The listing builds one solid part. Answer for the finished solid, in the listing's coordinates (mm). Face numbers are marked on the shaded views. A direction names the side the tool comes from. Give positions to 0.01 mm unless a question says otherwise; leave off trailing zeros. Write each loop counter-clockwise with the first axis right and the second up, starting at its lowest first coordinate (ties: lowest second). Pieces come first, ordered by that corner, then holes. Notation, with made-up numbers: M 85,27 L 116,27 A18 cw 116,45 Z; hole C -39.5,-23.75 d11. An arc over 180 degrees is marked long. Return JSON: item names as keys, results as strings.
from build123d import *

# Parameters (mm, degrees)
LINEAR_AUSTRAGEN_D_NN1_DEPTH    = 20
FASE1_SIZE                      = 1
SKIZZE2_R                       = 1.5
SCHNITT_LINEAR_AUSTRAGEN1_DEPTH = 10
SKIZZE3_R                       = 1.5
SCHNITT_LINEAR_AUSTRAGEN2_DEPTH = 10
SKIZZE4_R                       = 2.25
SCHNITT_LINEAR_AUSTRAGEN3_DEPTH = 10


with BuildPart() as part:
    # Skizze1 → Linear-Austragen-Dünn1 (new, symmetric)
    with BuildSketch(Plane.XY):
        Polygon((0, 10), (0, 0), (10, 0), (10, 1), (1, 1), (1, 10), align=None)
    extrude(amount=LINEAR_AUSTRAGEN_D_NN1_DEPTH, both=True)

    # Fase1
    fase1_edges = [part.edges().sort_by_distance(p)[0] for p in [
        (0.5, 10, 20),
        (0.5, 10, -20),
        (10, 0.5, -20),
        (10, 0.5, 20),
    ]]
    chamfer(fase1_edges, length=FASE1_SIZE)

    # Skizze2 → Schnitt-Linear austragen1 (cut)
    with BuildSketch(Plane(origin=(1, 0, 0), x_dir=(0, 0, -1), z_dir=(1, 0, 0))):
        with Locations(Location((-17.5, 6, 0), (0, 0, 90))):
            Circle(SKIZZE2_R)
        with Locations(Location((17.5, 6, 0), (0, 0, 90))):
            Circle(SKIZZE2_R)
    extrude(amount=-SCHNITT_LINEAR_AUSTRAGEN1_DEPTH, mode=Mode.SUBTRACT)

    # Skizze3 → Schnitt-Linear austragen2 (cut)
    with BuildSketch(Plane(origin=(0, 1, 0), x_dir=(1, 0, 0), z_dir=(0, 1, 0))):
        with Locations(Location((6, -11, 0), (0, 0, 270))):
            Circle(SKIZZE3_R)
        with Locations(Location((6, 11, 0), (0, 0, 270))):
            Circle(SKIZZE3_R)
    extrude(amount=-SCHNITT_LINEAR_AUSTRAGEN2_DEPTH, mode=Mode.SUBTRACT)

    # Skizze4 → Schnitt-Linear austragen3 (cut)
    with BuildSketch(Plane(origin=(0, 1, 0), x_dir=(1, 0, 0), z_dir=(0, 1, 0))):
        with Locations(Location((6, 0, 0), (0, 0, 270))):
            Circle(SKIZZE4_R)
    extrude(amount=-SCHNITT_LINEAR_AUSTRAGEN3_DEPTH, mode=Mode.SUBTRACT)


solid = part.part
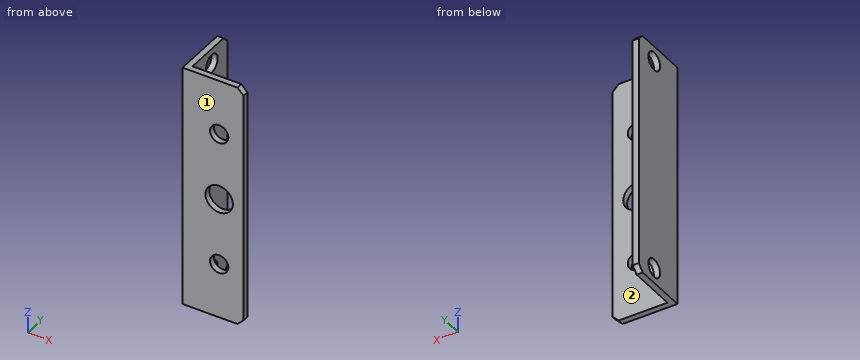
Item 1: A cutting plane is placed at A-A, the plane z = 0. Write down the section's boundary in (x, y).
Geometry results:
{"outline": "M 0,0 L 3.75,0 L 3.75,1 L 1,1 L 1,10 L 0,10 Z; M 8.25,0 L 10,0 L 10,1 L 8.25,1 Z"}
Item 2: A cutting plane is placed at C-C, the plane y = 6. Write down the section's boundary in (x, z).
Geometry results:
{"outline": "M 0,-20 L 1,-20 L 1,-19 L 0,-19 Z; M 0,-16 L 1,-16 L 1,16 L 0,16 Z; M 0,19 L 1,19 L 1,20 L 0,20 Z"}
Item 3: A cutting plane is placed at D-D, the plane z = 11. Write down the section's boundary in (x, y).
Geometry results:
{"outline": "M 0,0 L 4.5,0 L 4.5,1 L 1,1 L 1,10 L 0,10 Z; M 7.5,0 L 10,0 L 10,1 L 7.5,1 Z"}
Item 4: Which of the six approach directions +Z, -Z, +X, -X, +Y, -Y give full straight-line access (tool end or side, diameter ignored) to the marked faces 1 and 2?
Geometry results:
{"face 1": "+Z, -Z, +X, -X, -Y", "face 2": "+Z, -Z, +X, +Y"}
Item 5: A cutting plane is placed at B-B, the plane x = 6. Write down the section's boundary in (y, z), plus the area to 3 significant figures.
Geometry results:
{"outline": "M 0,-20 L 1,-20 L 1,-12.5 L 0,-12.5 Z; M 0,-9.5 L 1,-9.5 L 1,-2.25 L 0,-2.25 Z; M 0,2.25 L 1,2.25 L 1,9.5 L 0,9.5 Z; M 0,12.5 L 1,12.5 L 1,20 L 0,20 Z", "area": "29.5 mm2"}
Item 6: Find the intervals of material crossed by line 1 (Z direction, x = 0.4, y = 6); line 2 (X direction, y = 0.55, z = 11); line 3 (X direction, y = 0.75, z = 0), in increasing order.
Geometry results:
{"line 1": "z = -20 to -19, -16 to 16, 19 to 20", "line 2": "x = 0 to 4.5, 7.5 to 10", "line 3": "x = 0 to 3.75, 8.25 to 10"}
Item 7: Given pin 1 Ø2.5 at (x, z) = (6, 0) entering from -Y; pin 2 Ø4 at (y, z) = (6, 17.5) entering from +X; pin 3 Ø5 at (x, z) = (6, 11) entering from +Y, each flat-ended and moving along its own axis, determine where each tip first touches the part or whether it passes through.
Geometry results:
{"pin 1": "passes through", "pin 2": "stops at x = 1", "pin 3": "stops at y = 1"}
